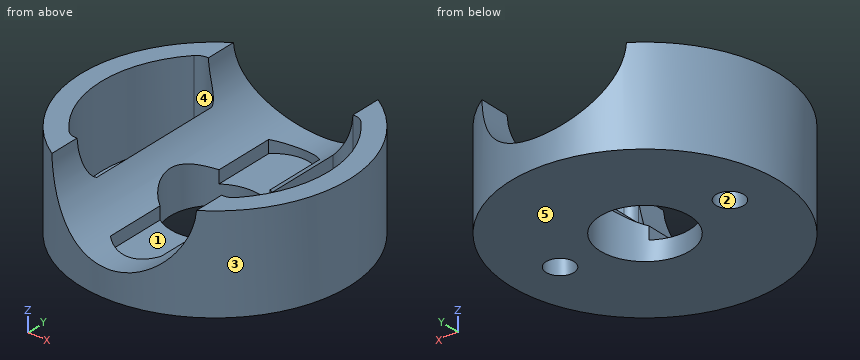
```python
from build123d import *

# Parameters (mm, degrees)
F1_DEPTH  = 15
F3_DEPTH  = 12
F5_DEPTH  = 9
F6_R      = 5
F7_DEPTH  = 12
F8_R      = 1.55
F9_DEPTH  = 12
F10_W     = 5.7
F10_H     = 22
F11_DEPTH = 3
F12_R     = 15
F12_R_2   = 1.55
F12_R_3   = 5
F13_DEPTH = 0.85


with BuildPart() as f1:
    # F0 (on Front) → F1 (new body, symmetric)
    with BuildSketch(Plane.XZ):
        with BuildLine():
            Line((-15, -6), (0, -6))
            Line((0, -6), (0, -2.1))
            ThreePointArc((0, -2.1), (-5.5691301799, 0.1182664936), (-8.0879356988, 5.5580767803))
            Line((-8.0879356988, 5.5580767803), (-15, 5.5580767803))
            Line((-15, 5.5580767803), (-15, -6))
        make_face()
        with BuildLine():
            Line((0, -6), (15, -6))
            Line((15, -6), (15, 5.5580767803))
            Line((15, 5.5580767803), (8.0879356988, 5.5580767803))
            ThreePointArc((8.0879356988, 5.5580767803), (5.5691301799, 0.1182664936), (0, -2.1))
            Line((0, -2.1), (0, -6))
        make_face()
    extrude(amount=F1_DEPTH, both=True)

    # F2 (on face) → F3 (cut)
    with BuildSketch(Plane.XY.offset(5.5580767803)):
        with BuildLine():
            Line((-8.0879356988, -15), (-8.0879356988, -12.6327073952))
            ThreePointArc((-8.0879356988, -12.6327073952), (-13.1590089963, -7.2000334884), (-15, 3.9e-09))
            Line((-15, 3.9e-09), (-15, -15))
            Line((-15, -15), (-8.0879356988, -15))
        make_face()
        with BuildLine():
            Line((-8.0879356988, -15), (0, -15))
            ThreePointArc((0, -15), (-4.2136319887, -14.396017), (-8.0879356988, -12.6327073952))
            Line((-8.0879356988, -12.6327073952), (-8.0879356988, -15))
        make_face()
        with BuildLine():
            ThreePointArc((-15, 3.9e-09), (-13.1590089945, 7.2000334918), (-8.0879356988, 12.6327073952))
            Line((-8.0879356988, 12.6327073952), (-8.0879356988, 15))
            Line((-8.0879356988, 15), (-15, 15))
            Line((-15, 15), (-15, 3.9e-09))
        make_face()
        with BuildLine():
            ThreePointArc((-8.0879356988, 12.6327073952), (-4.2136319887, 14.396017), (0, 15))
            Line((0, 15), (-8.0879356988, 15))
            Line((-8.0879356988, 15), (-8.0879356988, 12.6327073952))
        make_face()
        with BuildLine():
            ThreePointArc((0, 15), (10.6066017178, 10.6066017178), (15, 0))
            Line((15, 0), (15, 15))
            Line((15, 15), (0, 15))
        make_face()
        with BuildLine():
            Line((15, -15), (15, 0))
            ThreePointArc((15, 0), (10.6066017178, -10.6066017178), (0, -15))
            Line((0, -15), (15, -15))
        make_face()
    extrude(amount=-F3_DEPTH, mode=Mode.SUBTRACT)

    # F4 (on face) → F5 (cut)
    with BuildSketch(Plane.XY.offset(5.5580767803)):
        with BuildLine():
            ThreePointArc((-6.7912821949, 7.9907824623), (-7.8555088498, 9.0941072404), (-9.3332321619, 8.6863845995))
            ThreePointArc((-9.3332321619, 8.6863845995), (-12.75, 0), (-9.3332321619, -8.6863845995))
            ThreePointArc((-9.3332321619, -8.6863845995), (-7.8555088498, -9.0941072404), (-6.7912821949, -7.9907824623))
            Line((-6.7912821949, -7.9907824623), (-6.7912821949, 7.9907824623))
        make_face()
        with BuildLine():
            ThreePointArc((9.3332321619, -8.6863845995), (11.8651002959, -4.6671077733), (12.75, 0))
            ThreePointArc((12.75, 0), (11.8651002959, 4.6671077733), (9.3332321619, 8.6863845995))
            ThreePointArc((9.3332321619, 8.6863845995), (8.7631851378, 9.0573015192), (8.0879356988, 9.1383642487))
            Line((8.0879356988, 9.1383642487), (8.0879356988, -9.1383642487))
            ThreePointArc((8.0879356988, -9.1383642487), (8.7631851378, -9.0573015192), (9.3332321619, -8.6863845995))
        make_face()
        with BuildLine():
            Line((8.0879356988, -9.1383642487), (8.0879356988, 9.1383642487))
            ThreePointArc((8.0879356988, 9.1383642487), (7.2573018203, 8.7705623118), (6.7912821949, 7.9907824623))
            Line((6.7912821949, 7.9907824623), (6.7912821949, -7.9907824623))
            ThreePointArc((6.7912821949, -7.9907824623), (7.2573018203, -8.7705623118), (8.0879356988, -9.1383642487))
        make_face()
    extrude(amount=-F5_DEPTH, mode=Mode.SUBTRACT)

    # F6 (on face) → F7 (cut)
    with BuildSketch(Plane(origin=(0, 0, -6), x_dir=(1, 0, 0), z_dir=(0, 0, -1))):
        Circle(F6_R)
    extrude(amount=-F7_DEPTH, mode=Mode.SUBTRACT)

    # F8 (on face) → F9 (cut)
    with BuildSketch(Plane(origin=(0, 0, -6), x_dir=(1, 0, 0), z_dir=(0, 0, -1))):
        with Locations((-9.5, 0)):
            Circle(F8_R)
        with Locations((9.5, 0)):
            Circle(F8_R)
    extrude(amount=-F9_DEPTH, mode=Mode.SUBTRACT)

    # F10 (on Top) → F11 (cut)
    with BuildSketch(Plane.XY):
        Rectangle(F10_W, F10_H)
        with BuildLine():
            Line((-2.85, 11), (2.85, 11))
            ThreePointArc((2.85, 11), (0, 12.1933115599), (-2.85, 11))
        make_face()
        with BuildLine():
            ThreePointArc((-2.85, -11), (0, -12.1933115599), (2.85, -11))
            Line((2.85, -11), (-2.85, -11))
        make_face()
    extrude(amount=-F11_DEPTH, mode=Mode.SUBTRACT)

    # F12 (on face) → F13 (cut)
    with BuildSketch(Plane(origin=(0, 0, -6), x_dir=(1, 0, 0), z_dir=(0, 0, -1))):
        Circle(F12_R)
        with Locations((-9.5, 0)):
            Circle(F12_R_2, mode=Mode.SUBTRACT)
        Circle(F12_R_3, mode=Mode.SUBTRACT)
        with Locations((9.5, 0)):
            Circle(F12_R_2, mode=Mode.SUBTRACT)
    extrude(amount=-F13_DEPTH, mode=Mode.SUBTRACT)


solid = f1.part
```
For this review, take the finished solid that the model builds, in its own axes (mm). Face numbers are marked on the shaded views. A direction names the side the tool comes from. Coordinates: 2 decimals unless noted, no trailing zeros. Write each loop counter-clockwise with the first axis right and the second up, starting at its lowest first coordinate (ties: lowest second). Pieces come first, ordered by that corner, then holes.
(1) Add section C-C on y = -2.5. Give the boundary of the cut face in (x, z).
(2) Add section A-A on x = 0. Give the boundary of the cut face in (y, z).
(3) Tool access review of the marked faces 1 and 2: name each direction out of +Z, -Z, +X, -X, +Y, -Y from which nothing blocks a thin tool from reaching the whole face with its end or side.
(4) Add section B-B on z = 0. Give the boundary of the cut face in (x, y), then the cut area to 3 significant figures.
(5) For pin 1 Ø1 at (y, z) = (11.5, 1) entering from -X; pin 2 Ø1.6 at (y, z) = (7, -2.5) entering from +X; pin 3 Ø1.1 at (y, z) = (6, -2.5) entering from -X, all flat-tipped, find the tip position at first contact; note any pin that passes through.
(6) Add section D-D on y = 1. Give the boundary of the cut face in (x, z), then the cut area to 3 significant figures.
(7) Wall thickness on probe 1 along Y at (x, z) = (0, -3.6); probe 2 along X at (y, z) = (-4, -1); probe 3 along X at (y, z) = (6.5, -2.25): over which ranges is each line inside the solid? List them lowest first.
(8) The part is to be moulded in two halves that separate along Y. For the marked faces 3, 4 and 5, say which applies: +Y half, -Y half, draft (parallel to the pull), parting line (faces both ways), or undercut.
Answer sheet:
1. outline: (-14.79, -5.15) - (-4.33, -5.15) - (-4.33, -0.85) arc R8.1 cw to (-6.79, 1.59) - (-6.79, -3.44) - (-12.5, -3.44) - (-12.5, 5.56) - (-14.79, 5.56) - close; (4.33, -5.15) - (14.79, -5.15) - (14.79, 5.56) - (12.5, 5.56) - (12.5, -3.44) - (6.79, -3.44) - (6.79, 1.59) arc R8.1 cw to (4.33, -0.85) - close
2. outline: (-15, -5.15) - (-5, -5.15) - (-5, -3) - (-12.19, -3) - (-12.19, -2.1) - (-15, -2.1) - close; (5, -5.15) - (15, -5.15) - (15, -2.1) - (12.19, -2.1) - (12.19, -3) - (5, -3) - close
3. face 1: +Z
3. face 2: +Z, -Z
4. outline: (-5.44, -13.98) - (-5.44, 13.98) arc R15 ccw to start; (5.44, -13.98) arc R15 ccw to (5.44, 13.98) - close; hole (-9.33, -8.69) arc R1.5 ccw to (-6.79, -7.99) - (-6.79, 7.99) arc R1.5 ccw to (-9.33, 8.69) arc R12.75 ccw to start; hole (6.79, -7.99) arc R1.5 ccw to (9.33, -8.69) arc R12.75 ccw to (9.33, 8.69) arc R1.5 ccw to (6.79, 7.99) - close
4. area: 215 mm2
5. pin 1: stops at x = -10.2
5. pin 2: stops at x = 13.66
5. pin 3: stops at x = -13.97
6. outline: (-14.97, -5.15) - (-10.68, -5.15) - (-10.68, -3.44) - (-12.71, -3.44) - (-12.71, 5.56) - (-14.97, 5.56) - close; (-8.32, -5.15) - (-4.9, -5.15) - (-4.9, -0.45) arc R8.1 cw to (-6.79, 1.59) - (-6.79, -3.44) - (-8.32, -3.44) - close; (4.9, -5.15) - (8.32, -5.15) - (8.32, -3.44) - (6.79, -3.44) - (6.79, 1.59) arc R8.1 cw to (4.9, -0.45) - close; (10.68, -5.15) - (14.97, -5.15) - (14.97, 5.56) - (12.71, 5.56) - (12.71, -3.44) - (10.68, -3.44) - close
6. area: 81.6 mm2
7. probe 1: y = -15 to -5, 5 to 15
7. probe 2: x = -14.46 to -12.11, -6.79 to -4.08, 4.08 to 6.79, 12.11 to 14.46
7. probe 3: x = -13.52 to -10.97, -6.79 to -2.85, 2.85 to 6.79, 10.97 to 13.52
8. face 3: parting line
8. face 4: undercut
8. face 5: draft
